Check sheet for the modelled part. Datum: model origin and axes. Units: mm. A direction names the side the tool comes from. Round coordinates to 2 decimals unless told otherwise and drop trailing zeros. Write each loop counter-clockwise with the first axis right and the second up, starting at its lowest first coordinate (ties: lowest second). Pieces come first, ordered by that corner, then holes.
Item 1: Set-up check for faces 1 (the flat face through (11, -15, 0)), 2 (the flat face through (16, -2, 27.309)), 3 (the flat face through (24, 0, 0)), 4 (the flat face through (16, -2, -27.309)), 5 (the flat face through (-16, -2, -27.309)): record each of +Z, -Z, +X, -X, +Y, -Y from which the full face is reachable in a straight line by a thin tool's end or side.
Item 2: Release check for a two-part mould opening along Y. For faces 6 (the flat face through (-25, 0, 0)), 7 (the flat face through (-11, -15, 0)), 8 (the cylindrical face through (16.27, -32.22, 0.59)), 9 (the cylindrical face through (-16.13, -32.22, 0.59)) record: pulls with the +Y half, pulls with the -Y half, needs draft (parallel to the pull), parting line crosses it, or undercut.
Item 3: Section check B-B, the plane y = 5.5. Record the cut outline in (x, z).
Item 4: Section check C-C, the plane x = 0. Record the cut outline in (y, z), plus the area to 3 significant figures.
Item 5: Section check D-D, the plane y = -17. Record the cut outline in (x, z), plus the area to 3 significant figures.
Item 6: Depth check by flat-ended pin: pin 1 (6.5 mm diameter, centred on x = 25, z = -10, fed in from -Y); pin 2 (3 mm diameter, centred on x = -14, y = -34, fed in from -Z); pin 3 (4.5 mm diameter, centred on x = 0, z = 0, fed in from +Y); pin 4 (11.5 mm diameter, centred on x = 17.5, y = 3, fed in from -Z). Enter the tip coordinate at first touch or a pass-through.
Item 7: Section check A-A, the plane z = 0. Record the cut outline in (x, y).
Item 8: Material ranges on line 1 along X through (y, z) = (5.75, 0); line 2 along X through (y, z) = (-27, -12), recorded low to high.
from build123d import *

# Parameters (mm, degrees)
SKETCH1_R                = 29.440979716
BOSS_EXTRUDE1_DEPTH      = 10
SKETCH2_W                = 10.403384244
SKETCH2_H                = 54.617626702
BOSS_EXTRUDE2_DEPTH      = 40
BOSS_EXTRUDE2_DEPTH_BACK = 10
SKETCH3_R                = 2.7
CUT_EXTRUDE1_DEPTH       = 80
SKETCH4_R                = 2.7
CUT_EXTRUDE2_DEPTH       = 80
CUT_EXTRUDE2_DEPTH_BACK  = 80
SKETCH6_R                = 3
CUT_EXTRUDE3_DEPTH       = 80


with BuildPart() as part:
    # Sketch1 → Boss-Extrude1 (new body)
    with BuildSketch(Plane(origin=(0, 0, 0), x_dir=(1, 0, 0), z_dir=(0, 1, 0))):
        Circle(SKETCH1_R)
    extrude(amount=BOSS_EXTRUDE1_DEPTH)

    # Sketch2 → Boss-Extrude2 (add, two sides)
    with BuildSketch(Plane.XZ) as boss_extrude2_sk:
        with Locations((-16.201692122, 0)):
            Rectangle(SKETCH2_W, SKETCH2_H)
        with Locations((16.201692122, 0)):
            Rectangle(SKETCH2_W, SKETCH2_H)
    extrude(amount=BOSS_EXTRUDE2_DEPTH)
    extrude(boss_extrude2_sk.sketch, amount=-BOSS_EXTRUDE2_DEPTH_BACK)

    # Sketch3 → Cut-Extrude1 (cut)
    with BuildSketch(Plane(origin=(21.403384244, 0, 0), x_dir=(0, 0, -1), z_dir=(1, 0, 0))):
        with Locations((0, -29.584442491)):
            Circle(SKETCH3_R)
    extrude(amount=-CUT_EXTRUDE1_DEPTH, mode=Mode.SUBTRACT)

    # Sketch4 → Cut-Extrude2 (cut, two sides)
    with BuildSketch(Plane(origin=(0, 10, 0), x_dir=(1, 0, 0), z_dir=(0, 1, 0))) as cut_extrude2_sk:
        Circle(SKETCH4_R)
    extrude(amount=CUT_EXTRUDE2_DEPTH, mode=Mode.SUBTRACT)
    extrude(cut_extrude2_sk.sketch, amount=-CUT_EXTRUDE2_DEPTH_BACK, mode=Mode.SUBTRACT)

    # Cut-Sweep1: sweep along a path in Sketch5
    with BuildLine(Plane(origin=(0, 10, 0), x_dir=(1, 0, 0), z_dir=(0, 1, 0))) as cut_sweep1_path:
        CenterArc((0, 0), 15, 0, 360)
    # Sketch6 → Cut-Sweep1 (sweep, cut)
    with BuildSketch(Plane.XY):
        with Locations((-15, 10)):
            Circle(SKETCH6_R)
    sweep(path=cut_sweep1_path.line, mode=Mode.SUBTRACT)

    # Sketch8 → Cut-Extrude3 (cut)
    with BuildSketch(Plane.ZY.offset(21.403384244)):
        with BuildLine():
            Line((-27.308813351, -12.691186649), (-33.56023991, -12.691186649))
            Line((-33.56023991, -12.691186649), (-33.56023991, -51.85966326))
            Line((-33.56023991, -51.85966326), (31.545819747, -51.85966326))
            Line((31.545819747, -51.85966326), (31.545819747, -12.691186649))
            Line((31.545819747, -12.691186649), (27.308813351, -12.691186649))
            ThreePointArc((27.308813351, -12.691186649), (0, -40), (-27.308813351, -12.691186649))
        make_face()
    extrude(amount=-CUT_EXTRUDE3_DEPTH, mode=Mode.SUBTRACT)


solid = part.part
Values found:
1. face 1: +Z, -Z, -Y
1. face 2: +Z, +X, +Y, -Y
1. face 3: +Z, -Z, +X, -Y
1. face 4: -Z, +X, +Y, -Y
1. face 5: -Z, -X, +Y, -Y
2. face 6: pulls with the -Y half
2. face 7: needs draft
2. face 8: undercut
2. face 9: undercut
3. outline: (-21.4, -27.31) - (-11, -27.31) arc R29.44 ccw to (11, -27.31) - (21.4, -27.31) - (21.4, -20.22) arc R29.44 ccw to (21.4, 20.22) - (21.4, 27.31) - (11, 27.31) arc R29.44 ccw to (-11, 27.31) - (-21.4, 27.31) - (-21.4, 20.22) arc R29.44 ccw to (-21.4, -20.22) - close; hole circle Ø5.4 at (0, 0)
4. outline: (0, -29.44) - (10, -29.44) - (10, -18) arc R3 cw to (10, -12) - (10, -2.7) - (0, -2.7) - close; (0, 2.7) - (10, 2.7) - (10, 12) arc R3 cw to (10, 18) - (10, 29.44) - (0, 29.44) - close
4. area: 507 mm2
5. outline: (-21.4, -26.97) - (-11, -26.97) - (-11, 26.97) - (-21.4, 26.97) - close; (11, -26.97) - (21.4, -26.97) - (21.4, 26.97) - (11, 26.97) - close
5. area: 1,120 mm2
6. pin 1: stops at y = 0
6. pin 2: stops at z = -18.8
6. pin 3: passes through
6. pin 4: stops at z = -27.31
7. outline: (-29.44, 0) - (-21.4, 0) - (-21.4, -26.88) - (-11, -26.88) - (-11, 0) - (-2.7, 0) - (-2.7, 10) - (-12, 10) arc R3 cw to (-18, 10) - (-29.44, 10) - close; (-21.4, -40) - (-11, -40) - (-11, -32.28) - (-21.4, -32.28) - close; (2.7, 0) - (11, 0) - (11, -26.88) - (21.4, -26.88) - (21.4, 0) - (29.44, 0) - (29.44, 10) - (18, 10) arc R3 cw to (12, 10) - (2.7, 10) - close; (11, -40) - (21.4, -40) - (21.4, -32.28) - (11, -32.28) - close
8. line 1: x = -29.44 to -2.7, 2.7 to 29.44
8. line 2: x = -21.4 to -11, 11 to 21.4
